Design review of the part built by this model. Coordinates are the model's own, in mm. A direction names the side the tool comes from. Round coordinates to 2 decimals unless told otherwise and drop trailing zeros. Order: outer loops, then holes, each group sorted by start corner. A loop starts at its lowest first (then second) coordinate and runs counter-clockwise, first axis right, second up. Notation, with made-up numbers: (14, 48) - (67, 48) arc R19 cw to (67, 79) - close; hole circle Ø8 at (8.5, -12). An arc over 180 degrees is marked (long way). Use CSV: the item, a comma, the result in double quotes. Start each with the question number.
from build123d import *

# Parameters (mm, degrees)
SKETCH_1_W          = 48.6
SKETCH_1_H          = 42.6
EXTRUDE_1_DEPTH     = 3
SKETCH_2_W          = 48.6
SKETCH_2_H          = 42.6
SKETCH_2_W_2        = 40
SKETCH_2_H_2        = 35.6
EXTRUDE_2_DEPTH     = 7
SKETCH_3_W          = 20
SKETCH_3_H          = 4
SKETCH_3_W_2        = 38.6
SKETCH_3_H_2        = 3
EXTRUDE_3_DEPTH     = 20
SKETCH_6_W          = 15
SKETCH_6_H          = 3
SKETCH_6_W_2        = 5.7
SKETCH_6_H_2        = 4
EXTRUDE_4_DEPTH     = 5
SKETCH_7_W          = 5
SKETCH_7_H          = 12
EXTRUDE_5_DEPTH     = 20
SKETCH_8_R          = 0.95
CUT_EXTRUDE_1_DEPTH = 64.566107321
SKETCH_9_W          = 48.6
SKETCH_9_H          = 0.5
CUT_EXTRUDE_2_DEPTH = 0.5
SKETCH_10_W         = 0.5
SKETCH_10_H         = 42.6
CUT_EXTRUDE_3_DEPTH = 0.5


with BuildPart() as part:
    # 草图1 → 凸台-拉伸1 (new body)
    with BuildSketch(Plane(origin=(0, 0, 0), x_dir=(1, 0, 0), z_dir=(0, 1, 0))):
        Rectangle(SKETCH_1_W, SKETCH_1_H)
    extrude(amount=EXTRUDE_1_DEPTH)

    # 草图2 → 凸台-拉伸2 (add)
    with BuildSketch(Plane(origin=(0, 3, 0), x_dir=(1, 0, 0), z_dir=(0, 1, 0))):
        Rectangle(SKETCH_2_W, SKETCH_2_H)
        with Locations((0, 0.5)):
            Rectangle(SKETCH_2_W_2, SKETCH_2_H_2, mode=Mode.SUBTRACT)
    extrude(amount=EXTRUDE_2_DEPTH)

    # 草图3 → 凸台-拉伸3 (add)
    with BuildSketch(Plane(origin=(0, 10, 0), x_dir=(1, 0, 0), z_dir=(0, 1, 0))):
        with Locations((0, -19.3)):
            Rectangle(SKETCH_3_W, SKETCH_3_H)
        with Locations((0, 19.8)):
            Rectangle(SKETCH_3_W_2, SKETCH_3_H_2)
    extrude(amount=EXTRUDE_3_DEPTH)

    # 草图6 → 凸台-拉伸4 (add)
    with BuildSketch(Plane(origin=(0, 30, 0), x_dir=(1, 0, 0), z_dir=(0, 1, 0))):
        with Locations((-11.8, 19.8)):
            Rectangle(SKETCH_6_W, SKETCH_6_H)
        with Locations((11.8, 19.8)):
            Rectangle(SKETCH_6_W, SKETCH_6_H)
        with Locations((-7.15, -19.3)):
            Rectangle(SKETCH_6_W_2, SKETCH_6_H_2)
        with Locations((7.15, -19.3)):
            Rectangle(SKETCH_6_W_2, SKETCH_6_H_2)
    extrude(amount=EXTRUDE_4_DEPTH)

    # 草图7 → 凸台-拉伸5 (add)
    with BuildSketch(Plane(origin=(0, 3, 0), x_dir=(1, 0, 0), z_dir=(0, 1, 0))):
        with Locations((17.5, 12.3)):
            Rectangle(SKETCH_7_W, SKETCH_7_H)
        with Locations((-17.5, 12.3)):
            Rectangle(SKETCH_7_W, SKETCH_7_H)
    extrude(amount=EXTRUDE_5_DEPTH)

    # 草图8 → 切除-拉伸1 (cut, through all)
    with BuildSketch(Plane(origin=(24.3, 0, 0), x_dir=(0, 0, -1), z_dir=(1, 0, 0))):
        with Locations((13.3, 18)):
            Circle(SKETCH_8_R)
    extrude(amount=-CUT_EXTRUDE_1_DEPTH, mode=Mode.SUBTRACT)

    # 草图9 → 切除-拉伸2 (cut)
    with BuildSketch(Plane.XZ):
        with Locations((0, 11.05)):
            Rectangle(SKETCH_9_W, SKETCH_9_H)
        with Locations((0, -11.05)):
            Rectangle(SKETCH_9_W, SKETCH_9_H)
        Rectangle(SKETCH_9_W, SKETCH_9_H)
    extrude(amount=-CUT_EXTRUDE_2_DEPTH, mode=Mode.SUBTRACT)

    # 草图10 → 切除-拉伸3 (cut)
    with BuildSketch(Plane.XZ):
        Rectangle(SKETCH_10_W, SKETCH_10_H)
        with Locations((-14.05, 0)):
            Rectangle(SKETCH_10_W, SKETCH_10_H)
        with Locations((14.05, 0)):
            Rectangle(SKETCH_10_W, SKETCH_10_H)
    extrude(amount=-CUT_EXTRUDE_3_DEPTH, mode=Mode.SUBTRACT)


solid = part.part
Q1. The part is to be moulded in two halves that separate along Z. For faces 4 (the flat face through (0, 17, -21.3)), 5 (the flat face through (0, 15, 17.3)), 6 (the flat face through (19.3, 22, -20)), say which applies: +Z half, -Z half, draft (parallel to the pull), parting line (faces both ways), or undercut.
Q2. For L1, parallel to X at y = 13.5, z = -13.5; L2, parallel to X at y = 4, z = -9; L3, parallel to Y at x = 18.9, z = -13.3, list the stretches that pass through material, from the lowest coordinate up. Write a range as [from, to].
Q3. Take a section at A-A (y = 18). State the section outline as (x, z) points.
Q4. Take a section at B-B (z = -13.3). Give the number of separate pieces and of enclosed holes in the cut face, plus the area to 3 significant figures.
Q5. Take a section at D-D (x = 17). State the section outline as (y, z) points.
Q6. Clearance check with flat-ended pins moving along their axes: pin 1 (0.9 mm diameter, centred on x = -2, z = -19.5, fed in from +Y); pin 2 (12 mm diameter, centred on x = -9, z = 8.5, fed in from +Y); pin 3 (1.7 mm diameter, centred on y = 18, z = -13.3, fed in from -X); pin 4 (2 mm diameter, centred on y = 19.5, z = 20.5, fed in from +X). State where each tip first meets the part, or that it passes through.
Q7. Tool access review of faces 1 (the flat face through (15, 13, -12)), 2 (the flat face through (0, 30, -20)), 3 (the flat face through (-18, 23, -12)): name each direction out of +Z, -Z, +X, -X, +Y, -Y from which nothing blocks a thin tool from reaching the whole face with its end or side.
Q8. Take a section at C-C (y = 5). State the section outline as (x, z) points.
Findings below:
1,face 4,"-Z half"
1,face 5,"undercut"
1,face 6,"draft"
2,L1,"x = [-20, -15], [15, 20]"
2,L2,"x = [-24.3, -15], [15, 24.3]"
2,L3,"y = [0, 17.05], [18.95, 23]"
3,outline,"(-20, -18.3) - (-19.3, -18.3) - (-19.3, -21.3) - (19.3, -21.3) - (19.3, -18.3) - (20, -18.3) - (20, -14.25) - (15, -14.25) - (15, -18.3) - (-15, -18.3) - (-15, -14.25) - (-20, -14.25) - close; (-20, -12.35) - (-15, -12.35) - (-15, -6.3) - (-20, -6.3) - close; (-10, 17.3) - (10, 17.3) - (10, 21.3) - (-10, 21.3) - close; (15, -12.35) - (20, -12.35) - (20, -6.3) - (15, -6.3) - close"
4,separate pieces,"3"
4,enclosed holes,"0"
4,area,"386 mm^2"
5,outline,"(0, -21.3) - (35, -21.3) - (35, -18.3) - (23, -18.3) - (23, -6.3) - (3, -6.3) - (3, 17.3) - (10, 17.3) - (10, 21.3) - (0, 21.3) - (0, 11.3) - (0.5, 11.3) - (0.5, 10.8) - (0, 10.8) - (0, 0.25) - (0.5, 0.25) - (0.5, -0.25) - (0, -0.25) - (0, -10.8) - (0.5, -10.8) - (0.5, -11.3) - (0, -11.3) - close; hole circle Ø1.9 at (18, -13.3)"
6,pin 1,"stops at y = 30"
6,pin 2,"stops at y = 3"
6,pin 3,"passes through"
6,pin 4,"stops at x = 10"
7,face 1,"+Y"
7,face 2,"+Z, -Z, +Y"
7,face 3,"+Z, +X, -X, +Y"
8,outline,"(-24.3, -21.3) - (24.3, -21.3) - (24.3, 21.3) - (-24.3, 21.3) - close; hole (-20, -6.3) - (-15, -6.3) - (-15, -18.3) - (15, -18.3) - (15, -6.3) - (20, -6.3) - (20, 17.3) - (-20, 17.3) - close"
